from build123d import *

# Parameters (mm, degrees)
F1_DEPTH = 6.35
F3_DEPTH = 6.351
F4_R     = 9.525
F5_DEPTH = 6.351


with BuildPart() as f1:
    # F0 (on Top) → F1 (new body)
    with BuildSketch(Plane.XY):
        with BuildLine():
            ThreePointArc((82.55, 44.45), (78.830256, 53.430256), (69.85, 57.15))
            Line((69.85, 57.15), (-69.85, 57.15))
            ThreePointArc((-69.85, 57.15), (-78.830256, 53.430256), (-82.55, 44.45))
            Line((-82.55, 44.45), (-82.55, -44.45))
            ThreePointArc((-82.55, -44.45), (-78.830256, -53.430256), (-69.85, -57.15))
            Line((-69.85, -57.15), (69.85, -57.15))
            ThreePointArc((69.85, -57.15), (78.830256, -53.430256), (82.55, -44.45))
            Line((82.55, -44.45), (82.55, 44.45))
        make_face()
    extrude(amount=F1_DEPTH)

    # F2 (on face) → F3 (cut, through all)
    with BuildSketch(Plane.XY.offset(6.35)):
        with BuildLine():
            ThreePointArc((-69.85, -40.299123), (-71.925438, -42.374562), (-69.85, -44.45))
            Line((-69.85, -44.45), (-19.05, -44.45))
            ThreePointArc((-19.05, -44.45), (-16.974562, -42.374562), (-19.05, -40.299123))
            Line((-19.05, -40.299123), (-69.85, -40.299123))
        make_face()
        with BuildLine():
            Line((-19.05, -27.599123), (-69.85, -27.599123))
            ThreePointArc((-69.85, -27.599123), (-71.925438, -29.674562), (-69.85, -31.75))
            Line((-69.85, -31.75), (-19.05, -31.75))
            ThreePointArc((-19.05, -31.75), (-16.974562, -29.674562), (-19.05, -27.599123))
        make_face()
        with BuildLine():
            Line((-19.05, -14.899123), (-69.85, -14.899123))
            ThreePointArc((-69.85, -14.899123), (-71.925438, -16.974562), (-69.85, -19.05))
            Line((-69.85, -19.05), (-19.05, -19.05))
            ThreePointArc((-19.05, -19.05), (-16.974562, -16.974562), (-19.05, -14.899123))
        make_face()
        with BuildLine():
            Line((-19.05, -2.199123), (-69.85, -2.199123))
            ThreePointArc((-69.85, -2.199123), (-71.925438, -4.274562), (-69.85, -6.35))
            Line((-69.85, -6.35), (-19.05, -6.35))
            ThreePointArc((-19.05, -6.35), (-16.974562, -4.274562), (-19.05, -2.199123))
        make_face()
        with BuildLine():
            Line((-19.05, 10.500877), (-69.85, 10.500877))
            ThreePointArc((-69.85, 10.500877), (-71.925438, 8.425438), (-69.85, 6.35))
            Line((-69.85, 6.35), (-19.05, 6.35))
            ThreePointArc((-19.05, 6.35), (-16.974562, 8.425438), (-19.05, 10.500877))
        make_face()
        with BuildLine():
            Line((-19.05, 23.200877), (-69.85, 23.200877))
            ThreePointArc((-69.85, 23.200877), (-71.925438, 21.125438), (-69.85, 19.05))
            Line((-69.85, 19.05), (-19.05, 19.05))
            ThreePointArc((-19.05, 19.05), (-16.974562, 21.125438), (-19.05, 23.200877))
        make_face()
        with BuildLine():
            Line((-19.05, 35.900877), (-69.85, 35.900877))
            ThreePointArc((-69.85, 35.900877), (-71.925438, 33.825438), (-69.85, 31.75))
            Line((-69.85, 31.75), (-19.05, 31.75))
            ThreePointArc((-19.05, 31.75), (-16.974562, 33.825438), (-19.05, 35.900877))
        make_face()
        with BuildLine():
            Line((-19.05, 48.600877), (-69.85, 48.600877))
            ThreePointArc((-69.85, 48.600877), (-71.925438, 46.525438), (-69.85, 44.45))
            Line((-69.85, 44.45), (-19.05, 44.45))
            ThreePointArc((-19.05, 44.45), (-16.974562, 46.525438), (-19.05, 48.600877))
        make_face()
    extrude(amount=-F3_DEPTH, mode=Mode.SUBTRACT)

    # F4 (on face) → F5 (cut, through all)
    with BuildSketch(Plane.XY.offset(6.35)):
        with Locations((44.45, 0)):
            Circle(F4_R)
        with Locations((44.45, -31.75)):
            Circle(F4_R)
        with Locations((44.45, 31.75)):
            Circle(F4_R)
    extrude(amount=-F5_DEPTH, mode=Mode.SUBTRACT)


solid = f1.part
The model under review builds one solid part; all positions refer to its coordinate system, in mm. A direction names the side the tool comes from. Coordinates: 2 decimals unless noted, no trailing zeros. Loops run counter-clockwise (first coordinate to the right, second up) from the corner with the lowest first, then second, coordinate; pieces in that order, holes last. Notation, with made-up numbers: M -34,64 L -8,64 A27 cw -8,84 Z; hole C 74,11.5 d4. An arc over 180 degrees is marked long. Put each result on its own line as item: value. Start each with the question number.
Q1. Clearance check with a flat-ended pin moving along its axis: pin 1 (10 mm diameter, centred on x = -21, y = -15.5, fed in from -Z). State where the tip first meets the part, or that it passes through.
Q2. Add section C-C (y = 26.5). Write out the cut boundary in (x, z).
Q3. Add section A-A (y = 0). Write out the cut boundary in (x, z) (3 decimals), and give its area (3 significant figures).
Q4. Add section B-B (z = 1.75). Count the separate pieces of the cut face and the enclosed holes in it, and give its area (3 significant figures).
Q5. For faces 5 (the cylindrical face through (78.73, -53.53, 3.13)), 6 (the cylindrical face through (-16.975, -17.02, 3.219)), list the 3-axis set-ups (+Z, -Z, +X, -X, +Y, -Y) from which the entire face can be reached by the end or side of a thin tool; tool diameter is ignored.
Q6. The part is to be moulded in two halves that separate along X. For faces 1 (the flat face through (-44, 23.201, 3)), 2 (the flat face through (82.55, -1, 3)), 3 (the cylindrical face through (-78.93, -53.33, 3.13)), 4 (the flat face through (-45, -31.75, 3)), say which applies: +X half, -X half, draft (parallel to the pull), parting line (faces both ways), or undercut.
Q7. Wall thickness on line 1 (Y direction, x = 44.45, z = 4) (3 decimals); line 2 (X direction, y = 33.5, z = 3.5); line 3 (X direction, y = 35, z = 5.5): over which ranges is each line inside the solid? List them lowest first.
Answers:
1. pin 1: stops at z = 0
2. outline: M -82.55,0 L 36.5,0 L 36.5,6.35 L -82.55,6.35 Z; M 52.4,0 L 82.55,0 L 82.55,6.35 L 52.4,6.35 Z
3. outline: M -82.55,0 L 34.925,0 L 34.925,6.35 L -82.55,6.35 Z; M 53.975,0 L 82.55,0 L 82.55,6.35 L 53.975,6.35 Z
3. area: 927 mm^2
4. separate pieces: 1
4. enclosed holes: 11
4. area: 16,100 mm^2
5. face 5: +Z, -Z, +X, -Y
5. face 6: +Z, -Z
6. face 1: undercut
6. face 2: +X half
6. face 3: -X half
6. face 4: undercut
7. line 1: y = -57.15 to -41.275, -22.225 to -9.525, 9.525 to 22.225, 41.275 to 57.15
7. line 2: x = -82.55 to -71.9, -17 to 35.09, 53.81 to 82.55
7. line 3: x = -82.55 to -71.56, -17.34 to 35.5, 53.4 to 82.55
